from build123d import *

# Parameters (mm, degrees)
F1_DEPTH = 20
F2_R     = 1
F3_R     = 5
F3_W     = 5
F3_H     = 5
F4_DEPTH = 2.001
F5_R     = 5
F6_DEPTH = 2.001


with BuildPart() as f1:
    # F0 (on Front) → F1 (new body)
    with BuildSketch(Plane.XZ):
        with BuildLine():
            Line((0, 2), (0, 0))
            Line((0, 0), (27, 0))
            ThreePointArc((27, 0), (29.12132, 0.87868), (30, 3))
            Line((30, 3), (30, 30))
            Line((30, 30), (28, 30))
            Line((28, 30), (28, 3.5))
            ThreePointArc((28, 3.5), (27.56066, 2.43934), (26.5, 2))
            Line((26.5, 2), (0, 2))
        make_face()
    extrude(amount=F1_DEPTH)

    # F2
    f2_edges = [f1.edges().sort_by_distance(p)[0] for p in [
        (29, -20, 30),
        (29, 0, 30),
        (0, -20, 1),
        (0, 0, 1),
    ]]
    fillet(f2_edges, radius=F2_R)

    # F3 (on face) → F4 (cut, through all)
    with BuildSketch(Plane(origin=(28, 0, 0), x_dir=(0, -1, 0), z_dir=(-1, 0, 0))):
        with Locations((10, 20)):
            Circle(F3_R)
        with Locations((18.5, 7.5)):
            Rectangle(F3_W, F3_H)
    extrude(amount=-F4_DEPTH, mode=Mode.SUBTRACT)

    # F5 (on face) → F6 (cut, through all)
    with BuildSketch(Plane.XY.offset(2)):
        with Locations((10, -10)):
            Circle(F5_R)
    extrude(amount=-F6_DEPTH, mode=Mode.SUBTRACT)


solid = f1.part
Verification items for the finished model (mm, model axes). A direction names the side the tool comes from. Coordinates: 2 decimals unless noted, no trailing zeros. Order: outer loops, then holes, each group sorted by start corner. A loop starts at its lowest first (then second) coordinate and runs counter-clockwise, first axis right, second up. Notation, with made-up numbers: (-28, -16) -> (-19, -16) arc R16 ccw to (-19, -6) -> close; hole circle Ø6 at (-31, 31). An arc over 180 degrees is marked (long way). Use CSV: the item, a comma, the result in double quotes. Start each with the question number.
Q1. Depth check by flat-ended pin: P1, Ø6, axis at y = -11, z = 15, coming from the -X side; P2, Ø6, axis at y = -13.5, z = 6, coming from the -X side; P3, Ø1.6, axis at x = 29.5, z = 7, coming from the -Y side. Enter the tip coordinate at first touch or a pass-through.
Q2. Section check B-B, the plane x = 10. Record the cut outline in (y, z), and give its area (3 significant figures).
Q3. Tool access check on faces 4 (the flat face through (28, -10, 14)), 5 (the flat face through (29, -18, 5)), 6 (the flat face through (15, -20, 1)). Record the directions out of +Z, -Z, +X, -X, +Y, -Y that give a thin tool (end or side, any length) a straight path to the whole face; none if there is none.
Q4. Section check D-D, the plane z = 20. Record the cut outline in (x, y).
Q5. Section check A-A, the plane y = -10. Record the cut outline in (x, z), and give its area (3 significant figures).
Q6. Section check C-C, the plane y = -18.25. Record the cut outline in (x, z), and give its area (3 significant figures).
Q7. Draft check along Y on faces 1 (the flat face through (29, -10, 30)), 2 (the cylindrical face through (0.285, -19.699, 0.986)), 3 (the cylindrical face through (28.986, -12.307, 15.564)). Enter one of: +Y half, -Y half, draft (parallel to the pull), parting line (faces both ways), or undercut.
Q8. Thickness scan on line 1 along Y through (x, z) = (10, 1.1); line 2 along X through (y, z) = (-3, 26.5); line 3 along Z through (x, y) = (19.5, -3.25). Record the ranges inside material, lowest first.
Returned:
1,P1,"stops at x = 28"
1,P2,"stops at x = 27.91"
1,P3,"stops at y = -16"
2,outline,"(-20, 0) -> (-15, 0) -> (-15, 2) -> (-20, 2) -> close; (-5, 0) -> (0, 0) -> (0, 2) -> (-5, 2) -> close"
2,area,"20.0 mm^2"
3,face 4,"+Z, -X, +Y, -Y"
3,face 5,"+X, -X, -Y"
3,face 6,"+Z, -Z, +X, -X, -Y"
4,outline,"(28, -20) -> (30, -20) -> (30, -15) -> (28, -15) -> close; (28, -5) -> (30, -5) -> (30, 0) -> (28, 0) -> close"
5,outline,"(0, 0) -> (5, 0) -> (5, 2) -> (0, 2) -> close; (15, 0) -> (27, 0) arc R3 ccw to (30, 3) -> (30, 15) -> (28, 15) -> (28, 3.5) arc R1.5 cw to (26.5, 2) -> (15, 2) -> close; (28, 25) -> (30, 25) -> (30, 30) -> (28, 30) -> close"
5,area,"74.6 mm^2"
6,outline,"(0, 0) -> (27, 0) arc R3 ccw to (30, 3) -> (30, 5) -> (28, 5) -> (28, 3.5) arc R1.5 cw to (26.5, 2) -> (0, 2) -> close; (28, 10) -> (30, 10) -> (30, 30) -> (28, 30) -> close"
6,area,"105 mm^2"
7,face 1,"draft"
7,face 2,"-Y half"
7,face 3,"undercut"
8,line 1,"y = -20 to -15, -5 to 0"
8,line 2,"x = 28 to 30"
8,line 3,"z = 0 to 2"
